Study the drawing (mm; zero at the part's minimum x, y, z) and answer. A direction names the side the tool comes from. Give positions to 0.01 mm unless a question says otherwise; leave off trailing zeros. Write each loop counter-clockwise with the first axis right and the second up, starting at its lowest first coordinate (ties: lowest second). Pieces come first, ordered by that corner, then holes. Notation, with made-up numbers: (-9, -2) - (46, -2) arc R19 cw to (46, 21) - close; hole circle Ø9 at (-24, -36.5). An arc over 180 degrees is marked (long way). Answer as CSV lines item,"result".
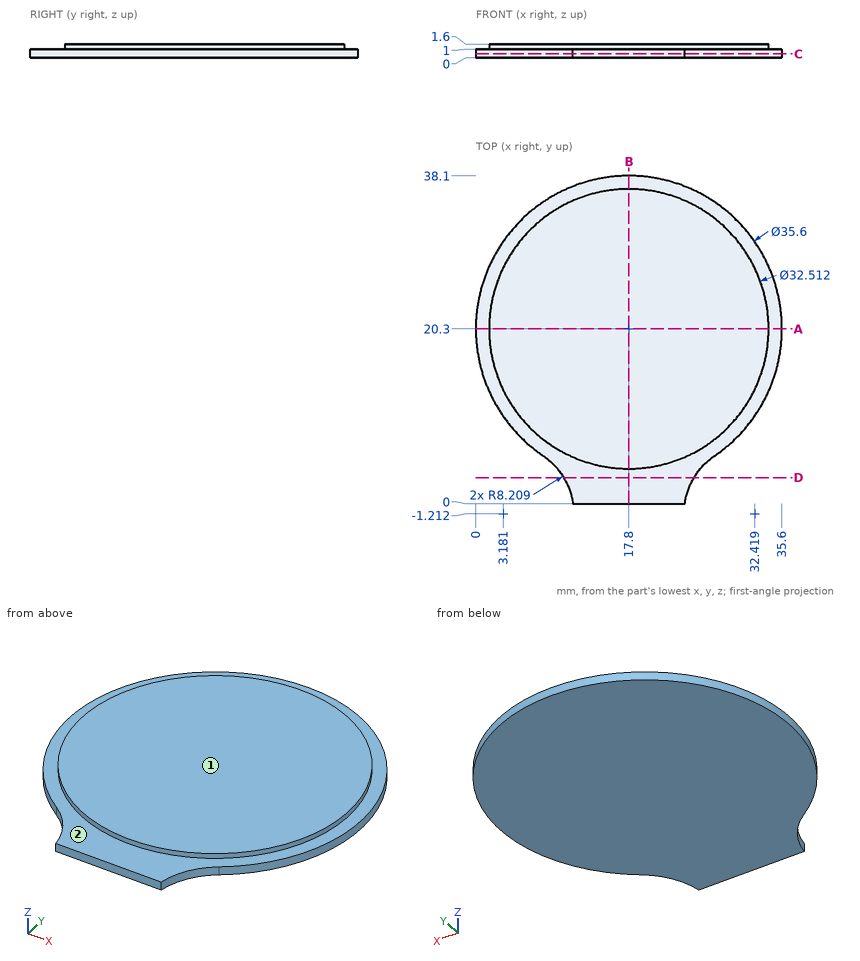
(1) Find the intervals of material crossed by L1, parallel to Z at x = 10, y = 36; L2, parallel to Y at x = 32, z = 0.25 (1 decimal); L3, parallel to Y at x = 14, z = 1.2 (1 decimal), in increasing order.
Worked out:
L1,"z = 0 to 1"
L2,"y = 9.6 to 31"
L3,"y = 4.5 to 36.1"
(2) A cutting plane is placed at D-D (y = 3). Write down the section's boundary in (x, z).
Worked out:
outline,"(10.23, 0) - (25.37, 0) - (25.37, 1) - (10.23, 1) - close"
(3) This flat-tipped pin is pushed along its axis until it touches: P1, Ø2, axis at x = 13.5, y = 24.5, coming from the -Z side. Where does it stop, or does it pass through?
Worked out:
P1,"stops at z = 0"
(4) A cutting plane is placed at B-B (x = 17.8). Write down the section's boundary in (y, z).
Worked out:
outline,"(0, 0) - (38.1, 0) - (38.1, 1) - (36.56, 1) - (36.56, 1.6) - (4.04, 1.6) - (4.04, 1) - (0, 1) - close"
(5) A cutting plane is placed at A-A (y = 20.3). Write down the section's boundary in (x, z).
Worked out:
outline,"(0, 0) - (35.6, 0) - (35.6, 1) - (34.06, 1) - (34.06, 1.6) - (1.54, 1.6) - (1.54, 1) - (0, 1) - close"
(6) For the marked faces 1 and 2, determine the directions among +Z, -Z, +X, -X, +Y, -Y from which every point of the face is accessible in a straight line to the end or side of a thin tool.
Worked out:
face 1,"+Z, +X, -X, +Y, -Y"
face 2,"+Z"
(7) A cutting plane is placed at C-C (z = 0.45). Write down the section's boundary in (x, y) (1 decimal).
Worked out:
outline,"(7.8, 5.6) arc R8.2 cw to (11.3, 0) - (24.3, 0) arc R8.2 cw to (27.8, 5.6) arc R17.8 ccw (long way) to start"
